from build123d import *

# Parameters (mm, degrees)
F0_W    = 1.6225828454
F0_H    = 6
F2_SIZE = 0.99999


# Not quite as in the source:
# - a fillet or chamfer is up to 0.001 mm smaller than in the source, because OpenCascade refuses the exact size


with BuildPart() as f1:
    # F0 (on Right) → F1 (revolve)
    with BuildSketch(Plane.YZ):
        Polygon((11, 6), (11, 0), (19.1040290039, 0), (19.1040290039, 9), (11, 9), (11, 7), align=None)
        with BuildLine():
            Line((19.1040290039, 9), (19.1040290039, 0))
            Line((19.1040290039, 0), (23, 0))
            ThreePointArc((23, 0), (21.9842102668, 4.9035341847), (19.1040290039, 9))
        make_face()
        Polygon((0, 7), (0, 0), (9.3774171546, 0), (9.3774171546, 6), (9.3774171546, 7), align=None)
        with Locations((10.1887085773, 3)):
            Rectangle(F0_W, F0_H)
    revolve(axis=Axis((0, 9.5520145019, 0), (0, 1, 0)))

    # F2 (size 1 in the source; OpenCascade refuses exactly that, so slightly less here)
    f2_edges = [f1.edges().sort_by_distance(p)[0] for p in [
        (0, 9.377417, -7),
        (0, 0, -7),
    ]]
    chamfer(f2_edges, length=F2_SIZE)


solid = f1.part
Model file for the job. Use its own axes, mm. A direction names the side the tool comes from. Give positions to 0.01 mm unless a question says otherwise; leave off trailing zeros. Loops run counter-clockwise (first coordinate to the right, second up) from the corner with the lowest first, then second, coordinate; pieces in that order, holes last.
1) Flat gauge pins, fed straight in: pin 1 Ø10 at (x, y) = (-4.5, 3.5) entering from -Z; pin 2 Ø3 at (x, y) = (-3, 16.5) entering from -Z; pin 3 Ø1.5 at (x, z) = (-4.5, 5.5) entering from +Y. Where does each tip first touch, or does it go through?
2) Pull direction Y, two halves, no side cores. Call faces 3 (the cylindrical face through (0, 10, -6)), 4 (the flat face through (0, 0, 0)), 5 (the cylindrical face through (-2.681, 4.637, 6.466)): +Y half, -Y half, draft (parallel to the pull), parting line (faces both ways), or undercut.
3) Saw through at B-B (y = 5.25). Write the cut outline in (x, z).
4) Tool access for faces 1 (the cylindrical face through (8.923, 14.995, -1.172)), 2 (the flat face through (-6, 11, 2)): list every direction of +Z, -Z, +X, -X, +Y, -Y with a clear straight run to the whole face (end or side of a thin tool).
5) Saw through at C-C (y = 15). Write the cut outline in (x, z), plus the area to 3 significant figures.
6) Wall check: line 1 (X direction, y = 4.75, z = 0.25); line 2 (Y direction, x = 0.75, z = 6.75); line 3 (Y direction, x = -6.5, z = -0.75). Give the ranges that are in metal, low to high.
Answer block:
1. pin 1: stops at z = -7
1. pin 2: stops at z = -8.87
1. pin 3: stops at y = 21.24
2. face 3: undercut
2. face 4: -Y half
2. face 5: draft
3. outline: circle Ø14 at (0, 0)
4. face 1: +Y, -Y
4. face 2: none
5. outline: circle Ø18 at (0, 0)
5. area: 254 mm2
6. line 1: x = -7 to 7
6. line 2: y = 0.79 to 8.59, 11 to 20.96
6. line 3: y = 0.54 to 8.83, 11 to 21.12
